Could you check a few things on this model? Use its own coordinates, in mm. A direction names the side the tool comes from. Round coordinates to 2 decimals unless told otherwise and drop trailing zeros. Write each loop counter-clockwise with the first axis right and the second up, starting at its lowest first coordinate (ties: lowest second). Pieces come first, ordered by that corner, then holes. Notation, with made-up numbers: (10.25, 64.25) -> (26.25, 64.25) arc R13 ccw to (26.25, 83.25) -> close; hole circle Ø2 at (67.5, -1). An arc over 180 degrees is marked (long way). Return JSON: item names as keys, results as strings.
from build123d import *

# Parameters (mm, degrees)
SKETCH1_W           = 33
SKETCH1_H           = 66
BOSS_EXTRUDE1_DEPTH = 8
SKETCH3_R           = 11.6
CUT_EXTRUDE1_DEPTH  = 62.269894728
SKETCH6_R           = 12.1
CUT_EXTRUDE2_DEPTH  = 5.1
SKETCH10_R          = 2.75
BOSS_EXTRUDE4_DEPTH = 7
CUT_EXTRUDE3_DEPTH  = 6
SKETCH12_R          = 2.75
CUT_EXTRUDE4_DEPTH  = 6
FILLET7_R           = 2
FILLET5_R           = 25
FILLET6_R           = 5.8
SKETCH13_R          = 3.5
SKETCH13_R_2        = 2.25
BOSS_EXTRUDE5_DEPTH = 8
FILLET8_R           = 2
CUT_EXTRUDE5_DEPTH  = 76.531450471


with BuildPart() as part:
    # Sketch1 → Boss-Extrude1 (new body)
    with BuildSketch(Plane.XY):
        with Locations((16.5, -18)):
            Rectangle(SKETCH1_W, SKETCH1_H)
    extrude(amount=BOSS_EXTRUDE1_DEPTH)

    # Sketch3 → Cut-Extrude1 (cut, through all)
    with BuildSketch(Plane.XY.offset(8)):
        Circle(SKETCH3_R)
    extrude(amount=-CUT_EXTRUDE1_DEPTH, mode=Mode.SUBTRACT)

    # Sketch6 → Cut-Extrude2 (cut)
    with BuildSketch(Plane(origin=(0, 0, 0), x_dir=(-1, 0, 0), z_dir=(0, 0, -1))):
        Circle(SKETCH6_R)
    extrude(amount=-CUT_EXTRUDE2_DEPTH, mode=Mode.SUBTRACT)

    # Sketch10 → Boss-Extrude4 (add)
    with BuildSketch(Plane.XZ.offset(51)):
        with BuildLine():
            Line((42, 0), (32, 0))
            Line((32, 0), (32, 10))
            ThreePointArc((32, 10), (49.071067812, 17.071067812), (42, 0))
        make_face()
        with Locations(Location((42, 10, 0), (0, 0, 270))):
            Circle(SKETCH10_R, mode=Mode.SUBTRACT)
    extrude(amount=-BOSS_EXTRUDE4_DEPTH)

    # Sketch11 → Cut-Extrude3 (cut)
    with BuildSketch(Plane.XY.offset(8)):
        with BuildLine():
            Line((0, -51), (24, -51))
            Line((24, -51), (24, -43))
            ThreePointArc((24, -43), (21.656854249, -37.343145751), (16, -35))
            Line((16, -35), (0, -35))
            Line((0, -35), (0, -51))
        make_face()
    extrude(amount=-CUT_EXTRUDE3_DEPTH, mode=Mode.SUBTRACT)

    # Sketch12 → Cut-Extrude4 (cut)
    with BuildSketch(Plane.XY.offset(2)):
        with Locations((8, -43)):
            Circle(SKETCH12_R)
    extrude(amount=-CUT_EXTRUDE4_DEPTH, mode=Mode.SUBTRACT)

    # Fillet7
    fillet7_edges = [part.edges().sort_by_distance(p)[0] for p in [
        (8, -35, 2),
        (21.656854249, -37.343145751, 2),
        (24, -47, 2),
    ]]
    fillet(fillet7_edges, radius=FILLET7_R)

    # Fillet5
    # the kernel refuses this fillet: 25 mm, written as the material it adds along each edge
    with BuildSketch(Plane(origin=(32, -44, 8), x_dir=(-1, 0, 0), z_dir=(0, -1, 0))) as fillet5_piece_1:
        with BuildLine():
            CenterArc((18.096713956, -22.870425604), FILLET5_R, 113.820244592, 29.574545381)
            Line((-1.972367441, -7.962978744), (-3.979275581, -6.472234058))
            ThreePointArc((-3.979275581, -6.472234058), (-2.5, -2), (-2.5, 0))
            Line((-2.5, 0), (0, 2.5))
            ThreePointArc((0, 2.5), (4, 2.5), (6.990328604, 2.28704256))
            Line((6.990328604, 2.28704256), (8, 0))
        make_face()
    extrude(amount=7)

    # Fillet6
    # the kernel refuses this fillet: 5.8 mm, written as the material it adds along each edge
    with BuildSketch(Plane(origin=(33, -44, 0), x_dir=(0, 1, 0), z_dir=(0, 0, 1))) as fillet6_piece_1:
        with BuildLine():
            CenterArc((FILLET6_R, -FILLET6_R), FILLET6_R, 90, 90)
            Line((0, -FILLET6_R), (0, 0))
            Line((0, 0), (FILLET6_R, 0))
        make_face()
    extrude(amount=8)
    with BuildSketch(Plane(origin=(33, -44, 8), x_dir=(0, 1, 0), z_dir=(-1, 0, 0))) as fillet6_piece_2_section:
        with BuildLine():
            CenterArc((FILLET6_R, -FILLET6_R), FILLET6_R, 90, 90)
            Line((0, -FILLET6_R), (0, 0))
            Line((0, 0), (FILLET6_R, 0))
        make_face()
    fillet6_piece_2 = extrude(amount=23.5, mode=Mode.PRIVATE)
    fillet6_piece_2 = fillet6_piece_2 - Plane(origin=(13.903286044, -44, 30.870425604), x_dir=(-1, 0, 0), z_dir=(0, 1, 0)) * Cylinder(25, 71, mode=Mode.PRIVATE)
    add(fillet6_piece_2)
    with BuildSketch(Plane(origin=(47.5, -44, 8), x_dir=(0, 1, 0), z_dir=(-1, 0, 0))) as fillet6_piece_3a_section:
        with BuildLine():
            CenterArc((FILLET6_R, -FILLET6_R), FILLET6_R, 90, 90)
            Line((0, -FILLET6_R), (0, 0))
            Line((0, 0), (FILLET6_R, 0))
        make_face()
    fillet6_piece_3a = extrude(amount=23.5, mode=Mode.PRIVATE)
    fillet6_piece_3a = fillet6_piece_3a - Plane(origin=(42, -44, 10), x_dir=(0, 0, -1), z_dir=(0, -1, 0)) * Cylinder(2.75, 71, mode=Mode.PRIVATE)
    fillet6_piece_3a = split(fillet6_piece_3a, bisect_by=Plane(origin=(33, -44, 8), z_dir=(1, 0, 0)), keep=Keep.TOP, mode=Mode.PRIVATE)
    with BuildSketch(Plane(origin=(33, -44, 0), x_dir=(0, 1, 0), z_dir=(0, 0, 1))) as fillet6_piece_3b_section:
        with BuildLine():
            CenterArc((FILLET6_R, -FILLET6_R), FILLET6_R, 90, 90)
            Line((0, -FILLET6_R), (0, 0))
            Line((0, 0), (FILLET6_R, 0))
        make_face()
    fillet6_piece_3b = extrude(amount=22.5, mode=Mode.PRIVATE)
    fillet6_piece_3b = split(fillet6_piece_3b, bisect_by=Plane(origin=(33, -44, 8), z_dir=(0, 0, 1)), keep=Keep.TOP, mode=Mode.PRIVATE)
    fillet6_piece_3b = fillet6_piece_3b & Plane(origin=(42, -44, 10), x_dir=(-1, 0, 0), z_dir=(0, -1, 0)) * Cylinder(10, 69, mode=Mode.PRIVATE)
    fillet6_piece_3 = fillet6_piece_3a & fillet6_piece_3b
    add(fillet6_piece_3)

    # Sketch13 → Boss-Extrude5 (add)
    with BuildSketch(Plane(origin=(0, 0, 0), x_dir=(-1, 0, 0), z_dir=(0, 0, -1))):
        with Locations((-8, -43)):
            Circle(SKETCH13_R)
        with Locations((-8, -43)):
            Circle(SKETCH13_R_2, mode=Mode.SUBTRACT)
    extrude(amount=-BOSS_EXTRUDE5_DEPTH)

    # Fillet8
    fillet8_edges = [part.edges().sort_by_distance(p)[0] for p in [
        (11.5, -43, 2),
    ]]
    fillet(fillet8_edges, radius=FILLET8_R)

    # Sketch15 → Cut-Extrude5 (cut, through all)
    with BuildSketch(Plane(origin=(0, 0, 0), x_dir=(-1, 0, 0), z_dir=(0, 0, -1))):
        with BuildLine():
            Line((0, 15), (-33, 15))
            Line((-33, 15), (-33, -3))
            ThreePointArc((-33, -3), (-29.485281374, 5.485281374), (-21, 9))
            ThreePointArc((-21, 9), (-14.200652085, 9.952282296), (-7.924528302, 12.735849057))
            ThreePointArc((-7.924528302, 12.735849057), (-4.120816918, 14.422859215), (0, 15))
        make_face()
    extrude(amount=-CUT_EXTRUDE5_DEPTH, mode=Mode.SUBTRACT)

    # Mirror1: part across plane


with BuildPart() as part_1:
    add(part.part)
    add(part.part.mirror(Plane(origin=(0, 15, 8), x_dir=(0, 0, 1), z_dir=(1, 0, 0))))


solid = part_1.part
1) Thinking about a two-plate mould opening in Y: for faces 6 (the face through (44.727, -47.549, 10.358)), 7 (the face through (8.46, -39.53, 5.97)), 8 (the face through (31.5, -42.3, 9.7)), which applies, pulls with the +Y half, pulls with the -Y half, needs draft (parallel to the pull), parting line crosses it, or undercut?
Return value:
{"face 6": "needs draft", "face 7": "undercut", "face 8": "pulls with the +Y half"}
2) I want a section at D-D, the plane x = -26. Please give me the cut outline in (y, z), and give its area (3 significant figures).
Return value:
{"outline": "(-51, 0) -> (7.91, 0) -> (7.91, 8) -> (-38.2, 8) arc R5.8 cw to (-41.44, 8.99) -> (-51, 8.99) -> close", "area": "482 mm²"}
3) If I drill on probe 1 along Z at (x, y) = (-42, -45.5); probe 2 along Z at (x, y) = (-25, 4.5); probe 3 along Y at (x, z) = (0, 1.8), over which ranges is the centre line in solid material (lowest first)? Write a range as [from, to].
Return value:
{"probe 1": "[0, 7.25], [12.75, 20]", "probe 2": "[0, 8]", "probe 3": "[-51, -12.1], [12.1, 15]"}
4) I want a section at B-B, the plane y = 5. Please give me the cut outline in (x, z).
Return value:
{"outline": "(-29.94, 0) -> (-11.02, 0) -> (-11.02, 5.1) -> (-10.47, 5.1) -> (-10.47, 8) -> (-29.94, 8) -> close; (10.47, 5.1) -> (11.02, 5.1) -> (11.02, 0) -> (29.94, 0) -> (29.94, 8) -> (10.47, 8) -> close"}
5) Will these pins go through, and if not, where does the flat tip stop? pin 1 Ø2 at (x, y) = (6.5, -41.5) entering from +Z; pin 2 Ø2 at (x, z) = (-1, 6) entering from -Y; pin 3 Ø6.5 at (y, z) = (-16.5, 3.5) entering from -X; pin 4 Ø2 at (y, z) = (-26.5, 10.5) entering from +X.
Return value:
{"pin 1": "z = 8", "pin 2": "y = -35", "pin 3": "x = -33", "pin 4": "through"}
6) For faces 1 (the face through (-33, -21, 4)), 2 (the face through (0, -35, 6)), 3 (the face through (29.58, 5.39, 3.94)), 4 (the face through (-23.4, -46.94, 2.57)), 5 (the face through (1, -51, 1)), which set-ups out of +Z, -Z, +X, -X, +Y, -Y let a thin tool reach every point of the face, with its end or its side?
Return value:
{"face 1": "+Z, -Z, -X, +Y", "face 2": "+Z", "face 3": "+Z, -Z, +X, +Y", "face 4": "+Z, -Y", "face 5": "+Z, -Z, +X, -X, -Y"}
7) I want a section at C-C, the plane z = 9. Please give me the cut outline in (x, y), and give its area (3 significant figures).
Return value:
{"outline": "(-51.95, -51) -> (-44.56, -51) -> (-44.56, -44) -> (-51.95, -44) -> close; (-39.44, -51) -> (-26.01, -51) -> (-26.01, -41.46) -> (-34, -41.46) arc R5.8 cw to (-38.8, -44) -> (-39.44, -44) -> close; (26.01, -51) -> (39.44, -51) -> (39.44, -44) -> (38.8, -44) arc R5.8 cw to (34, -41.46) -> (26.01, -41.46) -> close; (44.56, -51) -> (51.95, -51) -> (51.95, -44) -> (44.56, -44) -> close", "area": "339 mm²"}
8) I want a section at A-A, the plane x = 43.5. Please give me the cut outline in (y, z), and give its area (3 significant figures).
Return value:
{"outline": "(-51, 0.11) -> (-44, 0.11) -> (-44, 7.7) -> (-51, 7.7) -> close; (-51, 12.3) -> (-44, 12.3) -> (-44, 19.89) -> (-51, 19.89) -> close", "area": "106 mm²"}
